from build123d import *

# Parameters (mm, degrees)
SKETCH_W     = 54
SKETCH_H     = 31
SKETCH_W_2   = 50
SKETCH_H_2   = 27
PAD_DEPTH    = 4
PAD001_DEPTH = 2
PAD002_DEPTH = 2
PAD003_DEPTH = 2
PAD004_DEPTH = 2


with BuildPart() as part:
    # Sketch → Pad (new body)
    with BuildSketch(Plane.XY):
        with Locations((27, 15.5)):
            Rectangle(SKETCH_W, SKETCH_H)
        with Locations((27, 15.5)):
            Rectangle(SKETCH_W_2, SKETCH_H_2, mode=Mode.SUBTRACT)
    extrude(amount=PAD_DEPTH)

    # Sketch001 → Pad001 (join)
    with BuildSketch(Plane.XY):
        Polygon((2, 6), (6, 2), (2, 2), align=None)
    extrude(amount=PAD001_DEPTH)

    # Sketch002 → Pad002 (join)
    with BuildSketch(Plane.XY):
        Polygon((48, 29), (52, 25), (52, 29), align=None)
    extrude(amount=PAD002_DEPTH)

    # Sketch003 → Pad003 (join)
    with BuildSketch(Plane.XY):
        Polygon((2, 25), (6, 29), (2, 29), align=None)
    extrude(amount=PAD003_DEPTH)

    # Sketch004 → Pad004 (join)
    with BuildSketch(Plane.XY):
        Polygon((52, 6), (48, 2), (52, 2), align=None)
    extrude(amount=PAD004_DEPTH)


solid = part.part
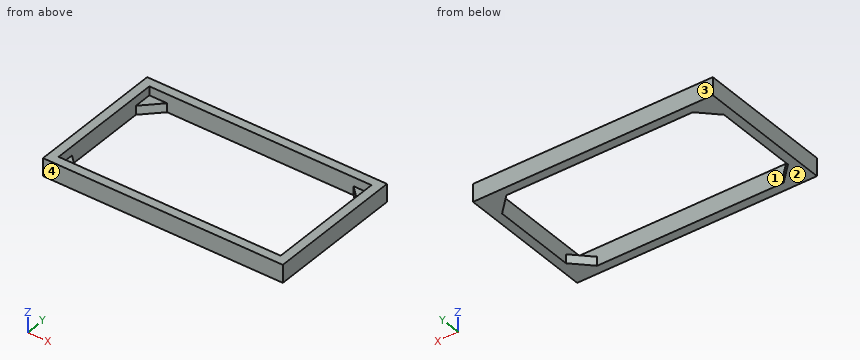
Design review of the part built by this model. Coordinates are the model's own, in mm. Face numbers are marked on the shaded views. Round coordinates to 2 decimals unless told otherwise and drop trailing zeros. Write each loop counter-clockwise with the first axis right and the second up, starting at its lowest first coordinate (ties: lowest second). Pieces come first, ordered by that corner, then holes. Notation, with made-up numbers: (13, 41) - (56, 41) arc R9 ccw to (56, 49) - close; hole circle Ø2 at (38.25, 11). An arc over 180 degrees is marked (long way). Return JSON: item names as keys, results as strings. Group by question number.
Item 1: The part is to be moulded in two halves that separate along Y. For the marked faces 1, 2, 3 and 4, say which applies: pulls with the +Y half, pulls with the -Y half, needs draft (parallel to the pull), parting line crosses it, or undercut.
Item 2: We need section A-A on x = 11. Write out the cut boundary in (y, z), and give its area (3 significant figures).
Item 3: We need section C-C on z = 0.85. Write out the cut boundary in (x, y), and give its area (3 significant figures).
Item 4: Insertion check: P1, Ø2, axis at x = 4, y = 27, coming from the +Z side. The pin has a flat end and moves straight along its axis. Give the tip position at first contact, or say it passes through.
Item 5: We need section D-D on x = 4. Write out the cut boundary in (y, z).
Item 6: We need section B-B on y = 22. Write out the cut boundary in (x, z), and give its area (3 significant figures).
Item 7: For probe 1 along X at (y, z) = (24, 3.35); probe 2 along Y at (x, z) = (5, 3.5); probe 3 along Y at (x, z) = (51.5, 0.5), list the stretches that pass through material, from the lowest coordinate up. Write a range as [from, to].
Model answer:
{
 "1": {"face 1": "undercut", "face 2": "needs draft", "face 3": "pulls with the +Y half", "face 4": "pulls with the -Y half"},
 "2": {"outline": "(0, 0) - (2, 0) - (2, 4) - (0, 4) - close; (29, 0) - (31, 0) - (31, 4) - (29, 4) - close", "area": "16.0 mm²"},
 "3": {"outline": "(0, 0) - (54, 0) - (54, 31) - (0, 31) - close; hole (2, 6) - (6, 2) - (48, 2) - (52, 6) - (52, 25) - (48, 29) - (6, 29) - (2, 25) - close", "area": "356 mm²"},
 "4": {"P1": "stops at z = 2"},
 "5": {"outline": "(0, 0) - (4, 0) - (4, 2) - (2, 2) - (2, 4) - (0, 4) - close; (27, 0) - (31, 0) - (31, 4) - (29, 4) - (29, 2) - (27, 2) - close"},
 "6": {"outline": "(0, 0) - (2, 0) - (2, 4) - (0, 4) - close; (52, 0) - (54, 0) - (54, 4) - (52, 4) - close", "area": "16.0 mm²"},
 "7": {"probe 1": "x = [0, 2], [52, 54]", "probe 2": "y = [0, 2], [29, 31]", "probe 3": "y = [0, 5.5], [25.5, 31]"}
}
